Here's how the part is built. I have some questions about the finished solid (model axes, mm). A direction names the side the tool comes from. Round coordinates to 2 decimals unless told otherwise and drop trailing zeros. Order: outer loops, then holes, each group sorted by start corner. A loop starts at its lowest first (then second) coordinate and runs counter-clockwise, first axis right, second up.
```python
from build123d import *

# Parameters (mm, degrees)
F0_W     = 20
F0_H     = 35
F1_DEPTH = 530
F2_W     = 25
F2_H     = 30
F3_DEPTH = 20
F4_R     = 2.5
F5_DEPTH = 25


with BuildPart() as f1:
    # F0 (on Front) → F1 (new body)
    with BuildSketch(Plane.XZ):
        Rectangle(F0_W, F0_H)
    extrude(amount=-F1_DEPTH)

    # F2 (on face) → F3 (cut)
    with BuildSketch(Plane.YZ.offset(10)):
        with Locations((12.5, 2.5)):
            Rectangle(F2_W, F2_H)
        with Locations((517.5, 2.5)):
            Rectangle(F2_W, F2_H)
    extrude(amount=-F3_DEPTH, mode=Mode.SUBTRACT)

    # F4 (on face) → F5 (cut)
    with BuildSketch(Plane.YZ.offset(10)):
        with Locations((55, 0)):
            Circle(F4_R)
        with Locations((480, 0)):
            Circle(F4_R)
    extrude(amount=-F5_DEPTH, mode=Mode.SUBTRACT)


solid = f1.part
```
1. If we section it at A-A, the plane x = 0: Write out the boundary of the cut face in (y, z).
Evaluation:
outline: (0, -17.5) - (530, -17.5) - (530, -12.5) - (505, -12.5) - (505, 17.5) - (25, 17.5) - (25, -12.5) - (0, -12.5) - close; hole circle Ø5 at (55, 0); hole circle Ø5 at (480, 0)
2. On a 3-axis mill with a long thin cutter (end or side, diameter ignored), from which of +Z, -Z, +X, -X, +Y, -Y can I reach the whole of each face in a straight line? I mean faces 1 (the flat face through (0, 517, -12.5)), 2 (the flat face through (-10, 261, 0)), 3 (the flat face through (0, 12, -12.5)). Say none if no direction works.
Evaluation:
face 1: +Z, +X, -X, +Y
face 2: +Z, -Z, -X, +Y, -Y
face 3: +Z, +X, -X, -Y
3. If we section it at B-B, the plane z = 7.5: Write out the boundary of the cut face in (x, y).
Evaluation:
outline: (-10, 25) - (10, 25) - (10, 505) - (-10, 505) - close
4. I need wall thicknesses on probe 1 along Z at (x, y) = (2, 55); probe 2 along Y at (x, z) = (3.5, -1); probe 3 along Y at (x, z) = (-3.5, 15). Which ranges of each line are inside material? Lowest first, please.
Evaluation:
probe 1: z = -17.5 to -2.5, 2.5 to 17.5
probe 2: y = 25 to 52.71, 57.29 to 477.71, 482.29 to 505
probe 3: y = 25 to 505
5. I'm going to push flat-ended pins straight in: P1, Ø10, axis at x = 4, y = 522, coming from the +Z side; P2, Ø10, axis at x = 4, z = -1, coming from the +Y side; P3, Ø12, axis at x = -6.5, z = -6, coming from the -Y side. Where does each tip first touch, or does it pass through?
Evaluation:
P1: stops at z = -12.5
P2: stops at y = 505
P3: stops at y = 25
